Build history of the part. All positions in model axes, mm. Round coordinates to 2 decimals unless told otherwise and drop trailing zeros. Write each loop counter-clockwise with the first axis right and the second up, starting at its lowest first coordinate (ties: lowest second). Pieces come first, ordered by that corner, then holes.
1) Pull direction X, two halves, no side cores. Call faces 1 (the flat face through (27.5, 13, 0)), 2 (the flat face through (-13.689, 0.493, 23.265)), 3 (the cylindrical face through (-16.855, 12.832, 2.213)): +X half, -X half, draft (parallel to the pull), parting line (faces both ways), or undercut.
2) Saw through at C-C (x = 23.5). Write the cut outline in (y, z), plus the area to 3 significant figures.
3) Saw through at B-B (y = 10). Write the cut outline in (x, z), plus the area to 3 significant figures.
4) Saw through at D-D (z = -27). Write the cut outline in (x, y).
5) Flat gauge pins, fed straight in: pin 1 (12 mm diameter, centred on x = -6, z = -5, fed in from +Y); pin 2 (4 mm diameter, centred on x = 8, y = 4, fed in from -Z); pin 3 (1.5 mm diameter, centred on x = 15, y = 16.5, fed in from -Z); pin 4 (3 mm diameter, centred on y = 12.5, z = -17.5, fed in from +X). Where does each tip first touch, or does it go through?
6) Saw through at A-A (z = 0). Write the cut outline in (x, y).
7) Wall check: probe 1 along X at (y, z) = (20.25, 0); probe 2 along Z at (x, y) = (13, 22.25); probe 3 along X at (y, z) = (12.75, -14.5). Give the ranges that are in metal, low to high.
from build123d import *

# Parameters (mm, degrees)
SKETCH_1_R      = 17
EXTRUDE_1_DEPTH = 26
CHAMFER_1_SIZE  = 1


with BuildPart() as part:
    # Эскиз1 → Бобышка-Вытянуть1 (new body)
    with BuildSketch(Plane(origin=(0, 0, 0), x_dir=(1, 0, 0), z_dir=(0, 1, 0))):
        Polygon((0, 31.754264805), (-27.5, 15.877132403), (-27.5, -15.877132403), (0, -31.754264805), (27.5, -15.877132403), (27.5, 15.877132403), align=None)
        with Locations(Location((0, 0, 0), (0, 0, 90))):
            Circle(SKETCH_1_R, mode=Mode.SUBTRACT)
    extrude(amount=EXTRUDE_1_DEPTH)

    # Фаска1
    chamfer_1_edges = [part.edges().sort_by_distance(p)[0] for p in [
        (-27.5, 26, 0),
        (-13.75, 26, 23.815698604),
        (0, 0, 17),
        (0, 26, 17),
        (13.75, 26, 23.815698604),
        (27.5, 26, 0),
        (13.75, 26, -23.815698604),
        (27.5, 0, 0),
        (13.75, 0, 23.815698604),
        (-13.75, 0, 23.815698604),
        (-27.5, 0, 0),
        (-13.75, 0, -23.815698604),
        (13.75, 0, -23.815698604),
        (-13.75, 26, -23.815698604),
    ]]
    chamfer(chamfer_1_edges, length=CHAMFER_1_SIZE)


solid = part.part
Evaluation:
1. face 1: +X half
1. face 2: -X half
1. face 3: undercut
2. outline: (0, -17.03) - (1, -18.19) - (25, -18.19) - (26, -17.03) - (26, 17.03) - (25, 18.19) - (1, 18.19) - (0, 17.03) - close
2. area: 943 mm2
3. outline: (-27.5, -15.88) - (0, -31.75) - (27.5, -15.88) - (27.5, 15.88) - (0, 31.75) - (-27.5, 15.88) - close; hole circle Ø34 at (0, 0)
3. area: 1,710 mm2
4. outline: (-8.23, 1) - (-6.23, 0) - (6.23, 0) - (8.23, 1) - (8.23, 25) - (6.23, 26) - (-6.23, 26) - (-8.23, 25) - close
5. pin 1: passes through
5. pin 2: stops at z = -28.29
5. pin 3: stops at z = -23.53
5. pin 4: stops at x = 27.29
6. outline: (-27.5, 1) - (-26.5, 0) - (-18, 0) - (-17, 1) - (-17, 25) - (-18, 26) - (-26.5, 26) - (-27.5, 25) - close; (17, 1) - (18, 0) - (26.5, 0) - (27.5, 1) - (27.5, 25) - (26.5, 26) - (18, 26) - (17, 25) - close
7. probe 1: x = -27.5 to -17, 17 to 27.5
7. probe 2: z = -24.25 to -10.95, 10.95 to 24.25
7. probe 3: x = -27.5 to -8.87, 8.87 to 27.5
